Geometry check sheet. Reference: the model listing, model coordinates, mm. A direction names the side the tool comes from. Round coordinates to 2 decimals unless told otherwise and drop trailing zeros. Write each loop counter-clockwise with the first axis right and the second up, starting at its lowest first coordinate (ties: lowest second). Pieces come first, ordered by that corner, then holes.
Item 1: Cross-section at A-A (z = 3.6). Enter the section's corners in (x, y).
Item 2: Cross-section at C-C (z = 0.6). Enter the section's corners in (x, y).
Item 3: Scan lines: probe 1 along Y at (x, z) = (0, 2.4); probe 2 along X at (y, z) = (1.5, 0.7); probe 3 along X at (y, z) = (-1.25, 3.8). Record each from-to range of solid material in increasing order.
Item 4: Depth check by flat-ended pin: P1, Ø1.5, axis at x = 6.5, z = 1.5, coming from the -Y side; P2, Ø1.5, axis at x = 4.5, z = 1.5, coming from the -Y side; P3, Ø1, axis at y = -3.5, z = 2, coming from the -X side. Enter the tip coordinate at first touch or a pass-through.
Item 5: Draft check along X on faces 3 (the face through (10.584, -3.923, 2.465)), 4 (the face through (-0.54, 2.44, 2.46)), 5 (the face through (9, 0, 0)). Enter one of: pulls with the +X half, pulls with the -X half, needs draft (parallel to the pull), parting line crosses it, or undercut.
Item 6: Access from +Z, -Z, +X, -X, +Y, -Y to the whole of each face (thin tool, end or side, straight path). Record for faces 1 (the face through (20.873, 1.049, 1.479)), 2 (the face through (15.82, 3.2, 4.01)).
Item 7: Cross-section at B-B (x = -1.5). Enter the section's corners in (y, z), then the cut area to 3 significant figures.
Item 8: Cross-section at D-D (y = 4.25). Enter the section's corners in (x, z).
Autodesk Inventor part; units mm, degrees
ref_plane "YZ Plane" through (0, 0, 0) normal (1, 0, 0) x (0, 1, 0)
ref_plane "XZ Plane" through (0, 0, 0) normal (0, 1, 0) x (-1, 0, 0)
ref_plane "XY Plane" through (0, 0, 0) normal (0, 0, 1) x (1, 0, 0)
sketch "Sketch1" plane through (0, 0, 0) normal (0, 0, 1) x (1, 0, 0)
  circle A0 centre (0, 0) radius 2.5
  circle A1 centre (0, 0) radius 5.5
  circle A2 centre (19.4422, 1.5) radius 1.5
  circle A3 centre (19.4422, 1.5) radius 4
  line L0 (0, 5.5) -> (19.4422, 5.5)
  line L1 (20.0558, -2.4527) -> (0.8436, -5.4349)
  point P0 (22.8922, -0.5243)
  dimension "d0" = 5
  dimension "d1" = 11
  dimension "d2" = 3
  dimension "d3" = 8
  dimension "d4" = 19.5
extrude "Extrusion1" add sketch "Sketch1" along normal blind 5
sketch "Sketch2" plane through (0, 0, 5) normal (0, 0, 1) x (1, 0, 0)
  circle A0 centre (19.4422, 1.5) radius 1.5
  line L0 (24.0473, 1.8553) -> (22.0525, -2.3105)
  line L1 (22.0525, -2.3105) -> (17.4474, -2.6658)
  line L2 (17.4474, -2.6658) -> (14.8371, 1.1447)
  line L3 (14.8371, 1.1447) -> (16.832, 5.3105)
  line L4 (16.832, 5.3105) -> (21.4371, 5.6658)
  line L5 (21.4371, 5.6658) -> (24.0473, 1.8553)
  line L6 (0, 0) -> (19.4422, 1.5)
  dimension "d7" = 8
extrude "Extrusion2" cut sketch "Sketch2" against normal blind 2
properties part number "TA07" material "ABS Plastic"
Resolved:
1. outline: (0, 5.5) arc R5.5 ccw (long way) to (0.84, -5.43) - (19.9, -2.48) - (17.45, -2.67) - (14.84, 1.14) - (16.83, 5.31) - (19.29, 5.5) - close; hole circle Ø5 at (0, 0)
2. outline: (0, 5.5) arc R5.5 ccw (long way) to (0.84, -5.43) - (20.06, -2.45) arc R4 ccw to (19.44, 5.5) - close; hole circle Ø5 at (0, 0); hole circle Ø3 at (19.44, 1.5)
3. probe 1: y = -5.5 to -2.5, 2.5 to 5.5
3. probe 2: x = -5.29 to -2, 2 to 17.94, 20.94 to 23.44
3. probe 3: x = -5.36 to -2.17, 2.17 to 16.48
4. P1: stops at y = -4.67
4. P2: stops at y = -4.98
4. P3: stops at x = -4.61
5. face 3: pulls with the +X half
5. face 4: undercut
5. face 5: needs draft
6. face 1: +Z, -Z
6. face 2: +Z, +X
7. outline: (-5.29, 0) - (-2, 0) - (-2, 5) - (-5.29, 5) - close; (2, 0) - (5.29, 0) - (5.29, 5) - (2, 5) - close
7. area: 32.9 mm2
8. outline: (-3.49, 0) - (22.35, 0) - (22.35, 3) - (16.32, 3) - (16.32, 5) - (-3.49, 5) - close
